Autodesk Inventor part; units mm, degrees
ref_plane "YZ Plane" through (0, 0, 0) normal (1, 0, 0) x (0, 1, 0)
ref_plane "XZ Plane" through (0, 0, 0) normal (0, 1, 0) x (-1, 0, 0)
ref_plane "XY Plane" through (0, 0, 0) normal (0, 0, 1) x (1, 0, 0)
sketch "Sketch1" plane through (0, 0, 0) normal (0, 0, 1) x (1, 0, 0)
  line L0 (0, 0) -> (30, 0) construction
  line L1 (0, -6) -> (30, -6)
  line L2 (30, 6) -> (0, 6)
  arc A0 (0, 6) -> (0, -6) centre (0, 0) ccw
  arc A1 (30, -6) -> (30, 6) centre (30, 0) ccw
  point P0 (15, 0)
  dimension "d0" = 12
  dimension "d1" = 30
extrude "Extrusion1" add sketch "Sketch1" along normal blind 3
sketch "Sketch2" plane through (0, 0, 3) normal (0, 0, 1) x (1, 0, 0)
  point P0 (0, 0)
  point P1 (0, 0)
hole "Hole1" at (0, 0, 3) direction (0, 0, -1) diameter 3 end through all
properties part number "Pancake_Reverse Weight" material "Aluminum 6061"
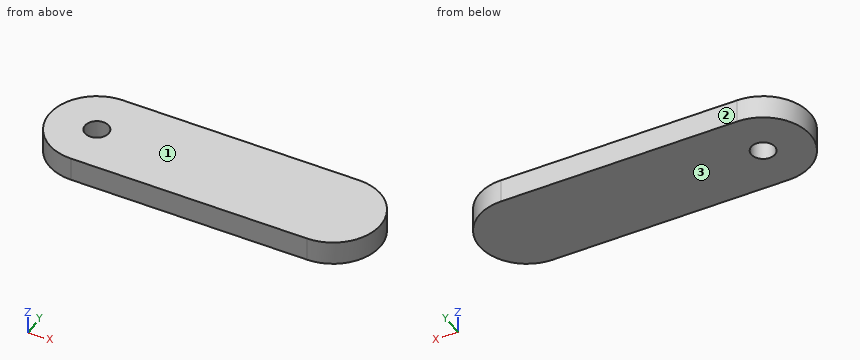
Here's how the part is built. I have some questions about the finished solid (model axes, mm). Face numbers are marked on the shaded views. Round coordinates to 2 decimals unless told otherwise and drop trailing zeros. Write each loop counter-clockwise with the first axis right and the second up, starting at its lowest first coordinate (ties: lowest second). Pieces come first, ordered by that corner, then holes.
Q1. If we section it at B-B on z = 1: Write out the boundary of the cut face in (x, y), plus the area to 3 significant figures.
Q2. If we mould it in two halves opening along Z, with no side actions, what happens to the marked faces 1, 2 and 3? For each: +Z half, -Z half, draft (parallel to the pull), parting line (faces both ways), or undercut.
Q3. Will this pin go through, and if not, where does the flat tip stop? P1, Ø1, axis at y = -2, z = 2, coming from the -X side.
Q4. Please list where these lines run through material, in increasing order: probe 1 along X at (y, z) = (0, 0.95); probe 2 along Y at (x, z) = (0, 0.8); probe 3 along X at (y, z) = (-1.25, 0.5).
Q5. If we section it at C-C on y = 2.25: Write out the boundary of the cut face in (x, z).
Q6. If we section it at A-A on y = 0: Write out the boundary of the cut face in (x, z), plus the area to 3 significant figures.
Answer below:
1. outline: (0, -6) - (30, -6) arc R6 ccw to (30, 6) - (0, 6) arc R6 ccw to start; hole circle Ø3 at (0, 0)
1. area: 466 mm2
2. face 1: +Z half
2. face 2: draft
2. face 3: -Z half
3. P1: stops at x = -5.81
4. probe 1: x = -6 to -1.5, 1.5 to 36
4. probe 2: y = -6 to -1.5, 1.5 to 6
4. probe 3: x = -5.87 to -0.83, 0.83 to 35.87
5. outline: (-5.56, 0) - (35.56, 0) - (35.56, 3) - (-5.56, 3) - close
6. outline: (-6, 0) - (-1.5, 0) - (-1.5, 3) - (-6, 3) - close; (1.5, 0) - (36, 0) - (36, 3) - (1.5, 3) - close
6. area: 117 mm2
